```python
from build123d import *

# Parameters (mm, degrees)
BOSS_EXTRUDE1_DEPTH = 9
CUT_EXTRUDE1_REACH  = 43.43
SKETCH2_R           = 2.25
FILLET1_R           = 2
FILLET2_R           = 1


with BuildPart() as part:
    # Sketch1 → Boss-Extrude1 (new body)
    with BuildSketch(Plane(origin=(0, 0, 0), x_dir=(1, 0, 0), z_dir=(0, 1, 0))):
        Polygon((8.212454023, 0), (0, 0), (-8.212454023, 0), (-18.115120739, -21.67), (-20.4, -26.67), (-14.902666716, -26.67), (-5, -5), (5, -5), (14.902666716, -26.67), (20.4, -26.67), (18.115120739, -21.67), align=None)
        Polygon((-20.4, -26.67), (-18.115120739, -21.67), (-30.4, -21.67), (-30.4, -26.67), align=None)
        Polygon((30.4, -21.67), (18.115120739, -21.67), (20.4, -26.67), (30.4, -26.67), align=None)
    extrude(amount=BOSS_EXTRUDE1_DEPTH)

    # Sketch2 → Cut-Extrude1 (cut, up to next)
    with BuildSketch(Plane.XY, mode=Mode.PRIVATE) as cut_extrude1_sk1:
        with Locations(Location((0, 4.5, 0), (0, 0, 180))):
            Circle(SKETCH2_R)
    cut_extrude1_tool1 = extrude(cut_extrude1_sk1.sketch, amount=CUT_EXTRUDE1_REACH, mode=Mode.PRIVATE) & part.part
    # Sketch2 → Cut-Extrude1 (cut, up to next)
    with BuildSketch(Plane.XY, mode=Mode.PRIVATE) as cut_extrude1_sk2:
        with Locations(Location((25.4, 4.5, 0), (0, 0, 180))):
            Circle(SKETCH2_R)
    cut_extrude1_tool2 = extrude(cut_extrude1_sk2.sketch, amount=CUT_EXTRUDE1_REACH, mode=Mode.PRIVATE) & part.part
    # Sketch2 → Cut-Extrude1 (cut, up to next)
    with BuildSketch(Plane.XY, mode=Mode.PRIVATE) as cut_extrude1_sk3:
        with Locations(Location((-25.4, 4.5, 0), (0, 0, 180))):
            Circle(SKETCH2_R)
    cut_extrude1_tool3 = extrude(cut_extrude1_sk3.sketch, amount=CUT_EXTRUDE1_REACH, mode=Mode.PRIVATE) & part.part
    add(cut_extrude1_tool1.solids().sort_by_distance((0, 4.5, 0))[0], mode=Mode.SUBTRACT)
    add(cut_extrude1_tool2.solids().sort_by_distance((25.4, 4.5, 0))[0], mode=Mode.SUBTRACT)
    add(cut_extrude1_tool3.solids().sort_by_distance((-25.4, 4.5, 0))[0], mode=Mode.SUBTRACT)

    # Fillet1
    fillet1_edges = [part.edges().sort_by_distance(p)[0] for p in [
        (-5, 4.5, 5),
        (-14.902666716, 4.5, 26.67),
        (-30.4, 4.5, 26.67),
        (-30.4, 4.5, 21.67),
        (-18.115120739, 4.5, 21.67),
        (-8.212454023, 4.5, 0),
        (8.212454023, 4.5, 0),
        (18.115120739, 4.5, 21.67),
        (30.4, 4.5, 21.67),
        (30.4, 4.5, 26.67),
        (14.902666716, 4.5, 26.67),
        (5, 4.5, 5),
    ]]
    fillet(fillet1_edges, radius=FILLET1_R)

    # Fillet2
    fillet2_edges = [part.edges().sort_by_distance(p)[0] for p in [
        (0, 0, 5),
        (0, 9, 5),
        (-9.951333358, 0, 15.835),
        (-9.951333358, 9, 15.835),
        (-22.293824163, 0, 26.67),
        (-30.4, 0, 24.17),
        (-23.900051174, 0, 21.67),
        (-13.163787381, 0, 10.835),
        (0, 0, 0),
        (13.163787381, 0, 10.835),
        (23.900051174, 0, 21.67),
        (30.4, 0, 24.17),
        (22.293824163, 0, 26.67),
        (9.951333358, 0, 15.835),
        (15.106569342, 0, 26.352637285),
        (29.814213562, 0, 26.084213562),
        (29.814213562, 0, 22.255786438),
        (8.008551397, 0, 0.317362715),
        (-8.008551397, 0, 0.317362715),
        (-29.814213562, 0, 22.255786438),
        (-29.814213562, 0, 26.084213562),
        (-15.106569342, 0, 26.352637285),
        (-22.293824163, 9, 26.67),
        (9.951333358, 9, 15.835),
        (22.293824163, 9, 26.67),
        (30.4, 9, 24.17),
        (23.900051174, 9, 21.67),
        (13.163787381, 9, 10.835),
        (0, 9, 0),
        (-13.163787381, 9, 10.835),
        (-23.900051174, 9, 21.67),
        (-30.4, 9, 24.17),
        (15.106569342, 9, 26.352637285),
        (29.814213562, 9, 26.084213562),
        (29.814213562, 9, 22.255786438),
        (8.008551397, 9, 0.317362715),
        (-8.008551397, 9, 0.317362715),
        (-29.814213562, 9, 22.255786438),
        (-29.814213562, 9, 26.084213562),
        (-15.106569342, 9, 26.352637285),
        (-4.796097374, 0, 5.317362715),
        (-4.796097374, 9, 5.317362715),
        (-18.319023366, 0, 21.352637285),
        (-18.319023366, 9, 21.352637285),
        (18.319023366, 0, 21.352637285),
        (18.319023366, 9, 21.352637285),
        (4.796097374, 0, 5.317362715),
        (4.796097374, 9, 5.317362715),
    ]]
    fillet(fillet2_edges, radius=FILLET2_R)


solid = part.part
```
Could you check a few things on this model? Use its own coordinates, in mm. A direction names the side the tool comes from. Round coordinates to 2 decimals unless told otherwise and drop trailing zeros. Write each loop counter-clockwise with the first axis right and the second up, starting at its lowest first coordinate (ties: lowest second). Pieces come first, ordered by that corner, then holes. Notation, with made-up numbers: M 6.5,-12.75 L 26.5,-12.75 A28 ccw 26.5,6.25 Z; hole C -16.75,20.5 d7. An arc over 180 degrees is marked long. Answer in a Markdown table with one row per item. Add a question column.
Q1. On a 3-axis mill with a long thin cutter (end or side, diameter ignored), from which of +Z, -Z, +X, -X, +Y, -Y can I reach the whole of each face in a straight line? I mean faces 5 (the flat face through (9.89, 4.45, 15.7)), 6 (the cylindrical face through (-10.163, 8.715, 15.575)), 7 (the flat face through (-23, 4, 21.67)), 8 (the flat face through (23, 4, 21.67)). Say none if no direction works.
Q2. Imagine slicing it at D-D (x = -24.5). Please give me the cut outline in (y, z), then the cut area to 3 significant figures.
Q3. Imagine slicing it at C-C (y = 4.5). Give the number of separate pieces and of enclosed holes in the cut face, then the cut area to 3 significant figures.
Q4. If we mould it in two halves opening along X, with no side actions, what happens to faces 1 (the cylindrical face through (8, 4.55, 0.31)), 2 (the flat face through (2, 3, 0)), 3 (the cylindrical face through (-8, 4.55, 0.31)), 4 (the cylindrical face through (10.287, 0.285, 15.845))? For each: +X half, -X half, draft (parallel to the pull), parting line (faces both ways), or undercut.
Q5. Will these pins go through, and if not, where does the flat tip stop? pin 1 Ø4 at (y, z) = (6.5, 21.5) entering from +X; pin 2 Ø12 at (x, z) = (2, 18.5) entering from -Y; pin 3 Ø2 at (y, z) = (3.5, 21.5) entering from +X; pin 4 Ø3 at (y, z) = (1.5, 19) entering from +X.
Q6. Imagine slicing it at B-B (x = 21). Please give me the cut outline in (y, z), then the cut area to 3 significant figures.
Q7. If I drill on line 1 (Y direction, x = 25.4, z = 23.75); line 2 (X direction, y = 4.5, z = 3.95); line 3 (Z direction, x = -21.5, y = 5.25), over which ranges is the centre line in solid material (lowest first)? Write a range as from..to.
Q8. Imagine slicing it at A-A (x = 0). Please give me the cut outline in (y, z), then the cut area to 3 significant figures.
Values:
| question | item | result |
|---|---|---|
| 1 | face 5 | +Z, +Y, -Y |
| 1 | face 6 | +Z, +Y |
| 1 | face 7 | -Z, -X, +Y, -Y |
| 1 | face 8 | -Z, +X, +Y, -Y |
| 2 | outline | M 0,22.67 A1 ccw 1,21.67 L 2.44,21.67 L 2.44,26.67 L 1,26.67 A1 ccw 0,25.67 Z; M 6.56,21.67 L 8,21.67 A1 ccw 9,22.67 L 9,25.67 A1 ccw 8,26.67 L 6.56,26.67 Z |
| 2 | area | 23.5 mm^2 |
| 3 | separate pieces | 4 |
| 3 | enclosed holes | 0 |
| 3 | area | 372 mm^2 |
| 4 | face 1 | +X half |
| 4 | face 2 | draft |
| 4 | face 3 | -X half |
| 4 | face 4 | undercut |
| 5 | pin 1 | x = 30.39 |
| 5 | pin 2 | through |
| 5 | pin 3 | x = 30.02 |
| 5 | pin 4 | x = 17.58 |
| 6 | outline | M 0,22.67 A1 ccw 1,21.67 L 8,21.67 A1 ccw 9,22.67 L 9,25.67 A1 ccw 8,26.67 L 1,26.67 A1 ccw 0,25.67 Z |
| 6 | area | 44.1 mm^2 |
| 7 | line 1 | 0..2.25, 6.75..9 |
| 7 | line 2 | -10.02..-2.25, 2.25..10.02 |
| 7 | line 3 | 21.67..26.67 |
| 8 | outline | M 0,1 A1 ccw 1,0 L 2.25,0 L 2.25,5 L 1,5 A1 ccw 0,4 Z; M 6.75,0 L 8,0 A1 ccw 9,1 L 9,4 A1 ccw 8,5 L 6.75,5 Z |
| 8 | area | 21.6 mm^2 |
